Model file for the job. Use its own axes, mm. Give positions to 0.01 mm unless a question says otherwise; leave off trailing zeros. Loops run counter-clockwise (first coordinate to the right, second up) from the corner with the lowest first, then second, coordinate; pieces in that order, holes last. Notation, with made-up numbers: (25, 33) - (46, 33) arc R27 ccw to (46, 66) - close; hole circle Ø2 at (41.5, -29). An arc over 180 degrees is marked (long way). Answer as CSV lines item,"result". Start each with the question number.
Item 1: Drill centre lines: L1, parallel to Y at x = 15.5, z = 4.1; L2, parallel to Y at x = 0, z = 1.4; L3, parallel to Y at x = -15, z = 4.25. Where is each one in solid material? Low to high. Write a range as from..to.
Item 2: Saw through at A-A on x = -15.5. Give the cut face in (y, z), plus the area to 3 significant figures.
Item 3: Pull direction X, two halves, no side cores. Call faces 1 (the cylindrical face through (0.59, 4.46, 2.96)), 2 (the flat face through (-21, 0, 3)), 3 (the flat face through (0, 21, 3)): pulls with the +X half, pulls with the -X half, needs draft (parallel to the pull), parting line crosses it, or undercut.
Item 4: Saw through at B-B on y = 0. Give the cut face in (x, z), plus the area to 3 significant figures.
Item 5: Saw through at C-C on z = 0.85. Give the cut face in (x, y), plus the area to 3 significant figures.
from build123d import *

# Parameters (mm, degrees)
SKETCH_1_W          = 42
SKETCH_1_H          = 42
EXTRUDE_1_DEPTH     = 6
SKETCH_2_R          = 1.5
CUT_EXTRUDE_1_DEPTH = 31.298514815
SKETCH_3_R          = 4.5
CUT_EXTRUDE_2_DEPTH = 31.298514815


with BuildPart() as part:
    # 草图1 → 凸台-拉伸1 (new body)
    with BuildSketch(Plane.XY):
        Rectangle(SKETCH_1_W, SKETCH_1_H)
    extrude(amount=EXTRUDE_1_DEPTH)

    # 草图2 → 切除-拉伸1 (cut, through all)
    with BuildSketch(Plane(origin=(0, 0, 0), x_dir=(-1, 0, 0), z_dir=(0, 0, -1))):
        with Locations((-15.5, 15.5)):
            Circle(SKETCH_2_R)
        with Locations((15.5, 15.5)):
            Circle(SKETCH_2_R)
        with Locations((15.5, -15.5)):
            Circle(SKETCH_2_R)
        with Locations((-15.5, -15.5)):
            Circle(SKETCH_2_R)
    extrude(amount=-CUT_EXTRUDE_1_DEPTH, mode=Mode.SUBTRACT)

    # 草图3 → 切除-拉伸2 (cut, through all)
    with BuildSketch(Plane(origin=(0, 0, 0), x_dir=(-1, 0, 0), z_dir=(0, 0, -1))):
        Circle(SKETCH_3_R)
    extrude(amount=-CUT_EXTRUDE_2_DEPTH, mode=Mode.SUBTRACT)


solid = part.part
Responses:
1,L1,"-21..-17, -14..14, 17..21"
1,L2,"-21..-4.5, 4.5..21"
1,L3,"-21..-16.91, -14.09..14.09, 16.91..21"
2,outline,"(-21, 0) - (-17, 0) - (-17, 6) - (-21, 6) - close; (-14, 0) - (14, 0) - (14, 6) - (-14, 6) - close; (17, 0) - (21, 0) - (21, 6) - (17, 6) - close"
2,area,"216 mm2"
3,face 1,"undercut"
3,face 2,"pulls with the -X half"
3,face 3,"needs draft"
4,outline,"(-21, 0) - (-4.5, 0) - (-4.5, 6) - (-21, 6) - close; (4.5, 0) - (21, 0) - (21, 6) - (4.5, 6) - close"
4,area,"198 mm2"
5,outline,"(-21, -21) - (21, -21) - (21, 21) - (-21, 21) - close; hole circle Ø3 at (-15.5, -15.5); hole circle Ø3 at (-15.5, 15.5); hole circle Ø9 at (0, 0); hole circle Ø3 at (15.5, -15.5); hole circle Ø3 at (15.5, 15.5)"
5,area,"1,670 mm2"
